```python
from build123d import *

# Parameters (mm, degrees)
BOSS_EXTRUDE1_DEPTH                            = 6.35
CHAMFER1_SIZE                                  = 6.6548
CHAMFER1_SIZE_2                                = 3.842150571
CSK_FOR_4_FLAT_HEAD_MACHINE_SCREW1_D           = 3.2639
CSK_FOR_4_FLAT_HEAD_MACHINE_SCREW1_CSINK_D     = 5.715
CSK_FOR_4_FLAT_HEAD_MACHINE_SCREW1_CSINK_ANGLE = 82
CSK_FOR_4_FLAT_HEAD_MACHINE_SCREW2_D           = 3.2639
CSK_FOR_4_FLAT_HEAD_MACHINE_SCREW2_CSINK_D     = 5.715
CSK_FOR_4_FLAT_HEAD_MACHINE_SCREW2_CSINK_ANGLE = 82
CSK_FOR_4_FLAT_HEAD_MACHINE_SCREW3_D           = 3.2639
CSK_FOR_4_FLAT_HEAD_MACHINE_SCREW3_CSINK_D     = 5.715
CSK_FOR_4_FLAT_HEAD_MACHINE_SCREW3_CSINK_ANGLE = 82


with BuildPart() as part:
    # Sketch1 → Boss-Extrude1 (new body)
    with BuildSketch(Plane(origin=(0, 0, 0), x_dir=(0, 0, -1), z_dir=(1, 0, 0))):
        Polygon((-39.465115344, -250.191197903), (165.84064038, 105.408802097), (559.54064038, 105.408802097), (559.54064038, -250.191197903), align=None)
    extrude(amount=BOSS_EXTRUDE1_DEPTH)

    # Chamfer1
    # the kernel refuses this chamfer: 6.6548, 3.842150571 mm, written as the material it takes off along each edge
    with BuildSketch(Plane(origin=(6.35, 105.408802097, -148.6241021), x_dir=(-0.9998132206222078, 0.019326765612699946, 0), z_dir=(0, 0, -1))) as chamfer1_piece_1:
        Polygon((CHAMFER1_SIZE * 0.999813220622, -CHAMFER1_SIZE * 0.0193267656127), (-CHAMFER1_SIZE_2 * 0.0193267656147, -CHAMFER1_SIZE_2 * 0.999813220727), (0, 0), align=None)
    extrude(amount=428.13307656, mode=Mode.SUBTRACT)

    # CSK for #4 Flat Head Machine Screw1 (through all)
    with Locations(Plane(origin=(0, 38.098802097, -546.84064038), x_dir=(0, 0, -1), z_dir=(-1, 0, 0))):
        with Locations((0, 0), (-317.5, -25.4), (0, 152.4)):
            CounterSinkHole(CSK_FOR_4_FLAT_HEAD_MACHINE_SCREW1_D / 2, CSK_FOR_4_FLAT_HEAD_MACHINE_SCREW1_CSINK_D / 2, counter_sink_angle=CSK_FOR_4_FLAT_HEAD_MACHINE_SCREW1_CSINK_ANGLE)

    # CSK for #4 Flat Head Machine Screw2 (through all)
    with Locations(Plane.ZY):
        with Locations((-543.66564038, 88.866651525), (-530.96564038, 88.866651525)):
            CounterSinkHole(CSK_FOR_4_FLAT_HEAD_MACHINE_SCREW2_D / 2, CSK_FOR_4_FLAT_HEAD_MACHINE_SCREW2_CSINK_D / 2, counter_sink_angle=CSK_FOR_4_FLAT_HEAD_MACHINE_SCREW2_CSINK_ANGLE)

    # CSK for #4 Flat Head Machine Screw3 (through all)
    with Locations(Plane(origin=(0, -224.791197903, -483.34064038), x_dir=(0, 0, -1), z_dir=(-1, 0, 0))):
        with Locations((0, 0), (-228.6, 0)):
            CounterSinkHole(CSK_FOR_4_FLAT_HEAD_MACHINE_SCREW3_D / 2, CSK_FOR_4_FLAT_HEAD_MACHINE_SCREW3_CSINK_D / 2, counter_sink_angle=CSK_FOR_4_FLAT_HEAD_MACHINE_SCREW3_CSINK_ANGLE)


solid = part.part
```
The listing builds one solid part. Answer for the finished solid, in the listing's coordinates (mm). Coordinates: 2 decimals unless noted, no trailing zeros. Write each loop counter-clockwise with the first axis right and the second up, starting at its lowest first coordinate (ties: lowest second). Pieces come first, ordered by that corner, then holes. Notation, with made-up numbers: (16.5, 85) -> (35.5, 85) arc R18 cw to (35.5, 115) -> close; hole circle Ø10 at (84, 75.25). An arc over 180 degrees is marked (long way). Write each question's results on one line, items separated by ' | '. Start each with the question number.
1) Straight lines are drawn through the part: probe 1 along Y at (x, z) = (0.5, -530); probe 2 along Y at (x, z) = (6.25, -348.5); probe 3 along Z at (x, y) = (0.5, -113.5). For each, find the intervals that lie inside material, in ascending order.
2) A cutting plane is placed at B-B (y = -72.5). Determine the outline of the cut face in (x, z), then the cut area to 3 significant figures.
3) A cutting plane is placed at C-C (z = -137.5). Determine the outline of the cut face in (x, y), then the cut area to 3 significant figures.
4) Flat-ended cylindrical pins translate along their axes: pin 1 Ø4 at (y, z) = (-114.3, -546.84) entering from -X; pin 2 Ø1.5 at (x, y) = (1, -162) entering from +Z; pin 3 Ø1 at (x, y) = (5, -82) entering from +Z. Find the tip coordinate at first contact, or state that the pin passes through.
5) A cutting plane is placed at A-A (x = 4.5). Determine the outline of the cut face in (y, z).
Values follow:
1) probe 1: -250.19 to 86.64, 91.09 to 104.94 | probe 2: -250.19 to 101.62 | probe 3: -559.54 to -549.13, -544.55 to -39.45
2) outline: (0, -559.54) -> (6.35, -559.54) -> (6.35, -63.12) -> (0, -63.12) -> close | area: 3,150 mm²
3) outline: (0, -250.19) -> (6.35, -250.19) -> (6.35, 56.32) -> (0, 56.32) -> close | area: 1,950 mm²
4) pin 1: x = 0.98 | pin 2: z = -11.02 | pin 3: z = -57.35
5) outline: (-250.19, -559.54) -> (102.63, -559.54) -> (102.63, -164.24) -> (-250.19, 39.47) -> close; hole circle Ø3.26 at (-224.79, -483.34); hole circle Ø3.26 at (-224.79, -254.74); hole circle Ø3.26 at (-114.3, -546.84); hole circle Ø3.26 at (38.1, -546.84); hole circle Ø3.26 at (63.5, -229.34); hole circle Ø3.26 at (88.87, -543.67); hole circle Ø3.26 at (88.87, -530.97)
